```python
from build123d import *

# Parameters (mm, degrees)
SKETCH1_W           = 136.525
SKETCH1_H           = 50.8
BOSS_EXTRUDE1_DEPTH = 1.27
SKETCH3_R           = 3.2639
CUT_EXTRUDE1_DEPTH  = 2.27
CHAMFER1_SIZE       = 3.175
FILLET1_R           = 1.27


with BuildPart() as part:
    # Sketch1 → Boss-Extrude1 (new body)
    with BuildSketch(Plane.XY):
        with Locations((68.2625, 25.4)):
            Rectangle(SKETCH1_W, SKETCH1_H)
    extrude(amount=BOSS_EXTRUDE1_DEPTH)

    # Sketch3 → Cut-Extrude1 (cut, through all)
    with BuildSketch(Plane.XY.offset(1.27)):
        with Locations((93.6625, 25.4)):
            Circle(SKETCH3_R)
        with Locations((42.8625, 25.4)):
            Circle(SKETCH3_R)
    extrude(amount=-CUT_EXTRUDE1_DEPTH, mode=Mode.SUBTRACT)

    # Chamfer1
    chamfer1_edges = [part.edges().sort_by_distance(p)[0] for p in [
        (0, 0, 0.635),
        (0, 50.8, 0.635),
        (136.525, 50.8, 0.635),
        (136.525, 0, 0.635),
    ]]
    chamfer(chamfer1_edges, length=CHAMFER1_SIZE)

    # Fillet1
    fillet1_edges = [part.edges().sort_by_distance(p)[0] for p in [
        (133.35, 0, 0.635),
        (3.175, 0, 0.635),
        (0, 47.625, 0.635),
        (0, 3.175, 0.635),
        (133.35, 50.8, 0.635),
        (3.175, 50.8, 0.635),
        (136.525, 3.175, 0.635),
        (136.525, 47.625, 0.635),
    ]]
    fillet(fillet1_edges, radius=FILLET1_R)


solid = part.part
```
The model under review builds one solid part; all positions refer to its coordinate system, in mm. Round coordinates to 2 decimals unless told otherwise and drop trailing zeros. Write each loop counter-clockwise with the first axis right and the second up, starting at its lowest first coordinate (ties: lowest second). Pieces come first, ordered by that corner, then holes. Notation, with made-up numbers: (-32, 5.5) - (-25, 5.5) arc R13 ccw to (-25, 13.5) - close; hole circle Ø10 at (44.5, 60). An arc over 180 degrees is marked (long way). Answer as CSV lines item,"result". Start each with the question number.
(1) Draft analysis for pull direction X (two halves, no side actions). For faces 1 (the cylindrical face through (45.976, 26.38, 0.644)), 2 (the flat face through (134.95, 1.6, 0.63)), 3 (the flat face through (1.605, 1.57, 0.626)), state which applies: pulls with the +X half, pulls with the -X half, needs draft (parallel to the pull), parting line crosses it, or undercut.
(2) We need section A-A on y = 25.4. State the section outline as (x, z) points (3 decimals), plus the area to 3 significant figures.
(3) To check wall thickness, follow line 1 (X direction, y = 25, z = 0.95) (3 decimals); line 2 (X direction, y = 24.5, z = 0.95) (3 decimals); line 3 (X direction, y = 3, z = 1.15). State the ranges of each line that lie inside material, in increasing order.
Worked answers:
1,face 1,"undercut"
1,face 2,"pulls with the +X half"
1,face 3,"pulls with the -X half"
2,outline,"(0, 0) - (39.599, 0) - (39.599, 1.27) - (0, 1.27) - close; (46.126, 0) - (90.399, 0) - (90.399, 1.27) - (46.126, 1.27) - close; (96.926, 0) - (136.525, 0) - (136.525, 1.27) - (96.926, 1.27) - close"
2,area,"157 mm²"
3,line 1,"0 to 39.623, 46.102 to 90.423, 96.902 to 136.525"
3,line 2,"0 to 39.725, 46 to 90.525, 96.8 to 136.525"
3,line 3,"0.21 to 136.31"
